The listing builds one solid part. Answer for the finished solid, in the listing's coordinates (mm). A direction names the side the tool comes from. Give positions to 0.01 mm unless a question says otherwise; leave off trailing zeros. Order: outer loops, then holes, each group sorted by start corner. A loop starts at its lowest first (then second) coordinate and runs counter-clockwise, first axis right, second up. Notation, with made-up numbers: (47.25, 2) - (61.25, 2) arc R17 cw to (61.25, 32) - close; hole circle Ø5 at (23, -5). An arc over 180 degrees is marked (long way). Answer as CSV lines item,"result". Start each with the question number.
1. Which of the six approach directions +Z, -Z, +X, -X, +Y, -Y give full straight-line access (tool end or side, diameter ignored) to faces 4 (the flat face through (-18, -25, 35)), 5 (the flat face through (5, -25, 32)), 6 (the flat face through (-18, -25, 40)), 7 (the flat face through (17, -25, 40))?
2. Consider line 1 along Z through (x, y) = (-11.5, -37.5); line 2 along X through (y, z) = (-45, 30.5). Determine where each line is inside the solid, lowest interval first. Write a range as [from, to].
3. Section B-B on y = -25 is taken. Give the vertices of the cut face in (x, z).
4. Flat-ended cylindrical pins translate along their axes: pin 1 (4 mm diameter, centred on y = -17.5, z = 31.5, fed in from -X); pin 2 (1.5 mm diameter, centred on y = -20.5, z = 32, fed in from +X); pin 3 (12.5 mm diameter, centred on x = -20, y = -29, fed in from +Z); pin 4 (2.5 mm diameter, centred on y = -26.5, z = 41.5, fed in from -X). Find the tip coordinate at first contact, or state that the pin passes through.
5. Section C-C on z = 42 is taken. Give the vertices of the cut face in (x, y).
6. Determine the mould class of faces 1 (the flat face through (-5, -25, 23)), 2 (the flat face through (30, -25, 27)), 3 (the flat face through (-18, -25, 15)) for opening direction Z: +Z half, -Z half, draft (parallel to the pull), parting line (faces both ways), or undercut.
7. Section A-A on x = 26.5 is taken. Give the vertices of the cut face in (y, z), and give its area (3 significant figures).
from build123d import *

# Parameters (mm, degrees)
F0_W     = 10
F0_H     = 5
F0_W_2   = 25
F1_DEPTH = 50


with BuildPart() as f1:
    # F0 (on Front) → F1 (new body)
    with BuildSketch(Plane.XZ):
        with Locations((0, 42.5)):
            Rectangle(F0_W, F0_H)
        with Locations((0, 37.5)):
            Rectangle(F0_W, F0_H)
        with Locations((-17.5, 37.5)):
            Rectangle(F0_W_2, F0_H)
        with Locations((17.5, 37.5)):
            Rectangle(F0_W_2, F0_H)
        with Locations((0, 32.5)):
            Rectangle(F0_W, F0_H)
        with Locations((0, 27.5)):
            Rectangle(F0_W, F0_H)
        with Locations((-17.5, 27.5)):
            Rectangle(F0_W_2, F0_H)
        with Locations((17.5, 27.5)):
            Rectangle(F0_W_2, F0_H)
        with Locations((0, 22.5)):
            Rectangle(F0_W, F0_H)
        with Locations((0, 17.5)):
            Rectangle(F0_W, F0_H)
        with Locations((-17.5, 17.5)):
            Rectangle(F0_W_2, F0_H)
        with Locations((17.5, 17.5)):
            Rectangle(F0_W_2, F0_H)
        with Locations((0, 12.5)):
            Rectangle(F0_W, F0_H)
    extrude(amount=F1_DEPTH)


solid = f1.part
Checks:
1,face 4,"-X, +Y, -Y"
1,face 5,"+X, +Y, -Y"
1,face 6,"+Z, -X, +Y, -Y"
1,face 7,"+Z, +X, +Y, -Y"
2,line 1,"z = [15, 20], [25, 30], [35, 40]"
2,line 2,"x = [-5, 5]"
3,outline,"(-30, 15) - (-5, 15) - (-5, 10) - (5, 10) - (5, 15) - (30, 15) - (30, 20) - (5, 20) - (5, 25) - (30, 25) - (30, 30) - (5, 30) - (5, 35) - (30, 35) - (30, 40) - (5, 40) - (5, 45) - (-5, 45) - (-5, 40) - (-30, 40) - (-30, 35) - (-5, 35) - (-5, 30) - (-30, 30) - (-30, 25) - (-5, 25) - (-5, 20) - (-30, 20) - close"
4,pin 1,"stops at x = -30"
4,pin 2,"stops at x = 5"
4,pin 3,"stops at z = 40"
4,pin 4,"stops at x = -5"
5,outline,"(-5, -50) - (5, -50) - (5, 0) - (-5, 0) - close"
6,face 1,"undercut"
6,face 2,"draft"
6,face 3,"-Z half"
7,outline,"(-50, 15) - (0, 15) - (0, 20) - (-50, 20) - close; (-50, 25) - (0, 25) - (0, 30) - (-50, 30) - close; (-50, 35) - (0, 35) - (0, 40) - (-50, 40) - close"
7,area,"750 mm²"
